from build123d import *

# Parameters (mm, degrees)
SKETCH_1_W                         = 2.79
SKETCH_1_H                         = 5
EXTRUDE_1_DEPTH                    = 8.4
SKETCH_2_W                         = 1
SKETCH_2_H                         = 1
CUT_EXTRUDE_1_DEPTH                = 8
CHAMFER_1_SIZE                     = 0.2
SKETCH_3_W                         = 0.64
SKETCH_3_H                         = 0.64
EXTRUDE_2_DEPTH                    = 2.29
CHAMFER_2_SIZE                     = 0.2
PATTERN_LINEAR_1_COUNT             = 3
PATTERN_LINEAR_1_PITCH             = 2.54
CHAMFER_1_OF_PATTERN_LINEAR_1_SIZE = 0.2
CHAMFER_2_OF_PATTERN_LINEAR_1_SIZE = 0.2


with BuildPart() as part:
    # Эскиз1 → Бобышка-Вытянуть1 (new body)
    with BuildSketch(Plane(origin=(0, 0, 0), x_dir=(1, 0, 0), z_dir=(0, 1, 0))):
        Rectangle(SKETCH_1_W, SKETCH_1_H)
    extrude_1 = extrude(amount=EXTRUDE_1_DEPTH)

    # Эскиз2 → Вырез-Вытянуть1 (cut)
    with BuildSketch(Plane(origin=(0, 8.4, 0), x_dir=(1, 0, 0), z_dir=(0, 1, 0))):
        with Locations((0, 1.27)):
            Rectangle(SKETCH_2_W, SKETCH_2_H)
        with Locations((0, -1.27)):
            Rectangle(SKETCH_2_W, SKETCH_2_H)
    cut_extrude_1 = extrude(amount=-CUT_EXTRUDE_1_DEPTH, mode=Mode.SUBTRACT)

    # Фаска1
    chamfer_1_edges = [part.edges().sort_by_distance(p)[0] for p in [
        (0.5, 8.4, -1.27),
        (0, 8.4, -1.77),
        (-0.5, 8.4, -1.27),
        (0, 8.4, -0.77),
        (0, 8.4, 1.77),
        (0.5, 8.4, 1.27),
        (0, 8.4, 0.77),
        (-0.5, 8.4, 1.27),
    ]]
    chamfer(chamfer_1_edges, length=CHAMFER_1_SIZE)

    # Эскиз3 → Бобышка-Вытянуть2 (add)
    with BuildSketch(Plane(origin=(0, 0, 0), x_dir=(-1, 0, 0), z_dir=(0, -1, 0))):
        with Locations((0, 1.27)):
            Rectangle(SKETCH_3_W, SKETCH_3_H)
        with Locations((0, -1.27)):
            Rectangle(SKETCH_3_W, SKETCH_3_H)
    extrude_2 = extrude(amount=EXTRUDE_2_DEPTH)

    # Фаска2
    chamfer_2_edges = [part.edges().sort_by_distance(p)[0] for p in [
        (0.32, -2.29, -1.27),
        (0, -2.29, -0.95),
        (-0.32, -2.29, -1.27),
        (0, -2.29, -1.59),
        (-0.32, -2.29, 1.27),
        (0, -2.29, 0.95),
        (0.32, -2.29, 1.27),
        (0, -2.29, 1.59),
    ]]
    chamfer(chamfer_2_edges, length=CHAMFER_2_SIZE)

    # Линейный массив1: Бобышка-Вытянуть1, Вырез-Вытянуть1, Бобышка-Вытянуть2 ×3
    with Locations(*[(i * PATTERN_LINEAR_1_PITCH, 0, 0) for i in range(1, PATTERN_LINEAR_1_COUNT)]):
        add(extrude_1)
        add(cut_extrude_1, mode=Mode.SUBTRACT)
        add(extrude_2)

    # Фаска1 of Линейный массив1
    chamfer_1_of_pattern_linear_1_edges = [part.edges().sort_by_distance(p)[0] for p in [
        (3.04, 8.4, -1.27),
        (2.54, 8.4, -1.77),
        (2.04, 8.4, -1.27),
        (2.54, 8.4, -0.77),
        (2.54, 8.4, 1.77),
        (3.04, 8.4, 1.27),
        (2.54, 8.4, 0.77),
        (2.04, 8.4, 1.27),
        (5.58, 8.4, -1.27),
        (5.08, 8.4, -1.77),
        (4.58, 8.4, -1.27),
        (5.08, 8.4, -0.77),
        (5.08, 8.4, 1.77),
        (5.58, 8.4, 1.27),
        (5.08, 8.4, 0.77),
        (4.58, 8.4, 1.27),
    ]]
    chamfer(chamfer_1_of_pattern_linear_1_edges, length=CHAMFER_1_OF_PATTERN_LINEAR_1_SIZE)

    # Фаска2 of Линейный массив1
    chamfer_2_of_pattern_linear_1_edges = [part.edges().sort_by_distance(p)[0] for p in [
        (2.86, -2.29, -1.27),
        (2.54, -2.29, -0.95),
        (2.22, -2.29, -1.27),
        (2.54, -2.29, -1.59),
        (2.22, -2.29, 1.27),
        (2.54, -2.29, 0.95),
        (2.86, -2.29, 1.27),
        (2.54, -2.29, 1.59),
        (5.4, -2.29, -1.27),
        (5.08, -2.29, -0.95),
        (4.76, -2.29, -1.27),
        (5.08, -2.29, -1.59),
        (4.76, -2.29, 1.27),
        (5.08, -2.29, 0.95),
        (5.4, -2.29, 1.27),
        (5.08, -2.29, 1.59),
    ]]
    chamfer(chamfer_2_of_pattern_linear_1_edges, length=CHAMFER_2_OF_PATTERN_LINEAR_1_SIZE)


solid = part.part
The listing builds one solid part. Answer for the finished solid, in the listing's coordinates (mm). A direction names the side the tool comes from. Round coordinates to 2 decimals unless told otherwise and drop trailing zeros. Loops run counter-clockwise (first coordinate to the right, second up) from the corner with the lowest first, then second, coordinate; pieces in that order, holes last. Notation, with made-up numbers: M -29,56.25 L -12,56.25 A28 cw -12,90.25 Z; hole C -21,51 d9. An arc over 180 degrees is marked long. Return JSON: item names as keys, results as strings.
Q1. Find the intervals of material crossed by line 1 along Z through (x, y) = (-0.25, 2); line 2 along X through (y, z) = (7.75, 1.5) (3 decimals); line 3 along Y through (x, z) = (1.25, -0.85), in increasing order. Write a range as from..to.
Results list:
{"line 1": "z = -2.5..-1.77, -0.77..0.77, 1.77..2.5", "line 2": "x = -1.395..-0.5, 0.5..2.04, 3.04..4.58, 5.58..6.475", "line 3": "y = 0..8.4"}
Q2. Find section B-B, the plane z = 0.25. Determine the outline of the cut face in (x, y) (3 decimals), plus the area to 3 significant figures.
Results list:
{"outline": "M -1.395,0 L 6.475,0 L 6.475,8.4 L -1.395,8.4 Z", "area": "66.1 mm2"}
Q3. Find section C-C, the plane x = 1.5. Determine the outline of the cut face in (y, z).
Results list:
{"outline": "M 0,-2.5 L 8.4,-2.5 L 8.4,2.5 L 0,2.5 Z"}
Q4. Each of these flat-tipped pins is pushed along its axis until it touches: pin 1 Ø0.5 at (y, z) = (-1.5, -1) entering from -X; pin 2 Ø0.5 at (y, z) = (-1, 1.5) entering from +X; pin 3 Ø0.7 at (x, y) = (5, -1.5) entering from -Z. Where does it stop, or does it pass through?
Results list:
{"pin 1": "stops at x = -0.32", "pin 2": "stops at x = 5.4", "pin 3": "stops at z = -1.59"}
Q5. Find section A-A, the plane y = 3. Determine the outline of the cut face in (x, z) (3 decimals).
Results list:
{"outline": "M -1.395,-2.5 L 6.475,-2.5 L 6.475,2.5 L -1.395,2.5 Z; hole M -0.5,-1.77 L 0.5,-1.77 L 0.5,-0.77 L -0.5,-0.77 Z; hole M -0.5,0.77 L 0.5,0.77 L 0.5,1.77 L -0.5,1.77 Z; hole M 2.04,-1.77 L 3.04,-1.77 L 3.04,-0.77 L 2.04,-0.77 Z; hole M 2.04,0.77 L 3.04,0.77 L 3.04,1.77 L 2.04,1.77 Z; hole M 4.58,-1.77 L 5.58,-1.77 L 5.58,-0.77 L 4.58,-0.77 Z; hole M 4.58,0.77 L 5.58,0.77 L 5.58,1.77 L 4.58,1.77 Z"}
Q6. Which of the six approach directions +Z, -Z, +X, -X, +Y, -Y give full straight-line access (tool end or side, diameter ignored) to faces 1 (the face through (0.5, 4, 1)), 2 (the face through (2, 4, 2.5))?
Results list:
{"face 1": "+Y", "face 2": "+Z, +X, -X, +Y, -Y"}
Q7. The mould has two halves that part along Z. Classify faces 3 (the face through (0, 0.4, -1)), 4 (the face through (-1.395, 4, 0)), 5 (the face through (2, 4, -2.5)): released by +Z, released by -Z, zero draft, split by the parting line, or undercut.
Results list:
{"face 3": "undercut", "face 4": "zero draft", "face 5": "released by -Z"}
